Can you work these out from the model? Positions are in its coordinate system, mm. A direction names the side the tool comes from. Give positions to 0.01 mm unless a question says otherwise; leave off trailing zeros. Loops run counter-clockwise (first coordinate to the right, second up) from the corner with the lowest first, then second, coordinate; pieces in that order, holes last. Notation, with made-up numbers: M -19.75,78 L -9.75,78 A12 ccw -9.75,101 Z; hole C -34.75,38 d1. An arc over 180 degrees is marked long. Use CSV: the item, a comma, the result in double quotes.
from build123d import *

# Parameters (mm, degrees)
F1_R           = 1.75
F2_DEPTH       = 5
F3_R           = 1.75
F4_DEPTH       = 5
F6_R           = 25
F7_DEPTH       = 5.001
F9_D           = 3.3
F9_CSINK_D     = 6.72
F9_CSINK_ANGLE = 90
F10_R          = 1.75
F11_DEPTH      = 2.5


with BuildPart() as f2:
    # F1 (on Top) → F2 (new body)
    with BuildSketch(Plane.XY):
        with BuildLine():
            Line((-1.4142135624, 41.0121933088), (-41.0121933088, 1.4142135624))
            ThreePointArc((-41.0121933088, 1.4142135624), (-41.5979797464, 0), (-41.0121933088, -1.4142135624))
            Line((-41.0121933088, -1.4142135624), (-1.4142135624, -41.0121933088))
            ThreePointArc((-1.4142135624, -41.0121933088), (0, -41.5979797464), (1.4142135624, -41.0121933088))
            Line((1.4142135624, -41.0121933088), (41.0121933088, -1.4142135624))
            ThreePointArc((41.0121933088, -1.4142135624), (41.5979797464, 0), (41.0121933088, 1.4142135624))
            Line((41.0121933088, 1.4142135624), (1.4142135624, 41.0121933088))
            ThreePointArc((1.4142135624, 41.0121933088), (0, 41.5979797464), (-1.4142135624, 41.0121933088))
        make_face()
        with Locations((0, -35.3553390593)):
            Circle(F1_R, mode=Mode.SUBTRACT)
        with Locations((-35.3553390593, 0)):
            Circle(F1_R, mode=Mode.SUBTRACT)
        with Locations((35.3553390593, 0)):
            Circle(F1_R, mode=Mode.SUBTRACT)
        with Locations((0, 35.3553390593)):
            Circle(F1_R, mode=Mode.SUBTRACT)
    extrude(amount=F2_DEPTH)


with BuildPart() as f4:
    # F3 (on Top) → F4 (new body)
    with BuildSketch(Plane.XY):
        with BuildLine():
            Line((23, 25), (-23, 25))
            ThreePointArc((-23, 25), (-24.4142135624, 24.4142135624), (-25, 23))
            Line((-25, 23), (-25, -23))
            ThreePointArc((-25, -23), (-24.4142135624, -24.4142135624), (-23, -25))
            Line((-23, -25), (23, -25))
            ThreePointArc((23, -25), (24.4142135624, -24.4142135624), (25, -23))
            Line((25, -23), (25, 23))
            ThreePointArc((25, 23), (24.4142135624, 24.4142135624), (23, 25))
        make_face()
        with Locations((-20, -20)):
            Circle(F3_R, mode=Mode.SUBTRACT)
        with Locations((20, -20)):
            Circle(F3_R, mode=Mode.SUBTRACT)
        with Locations((-20, 20)):
            Circle(F3_R, mode=Mode.SUBTRACT)
        with Locations((20, 20)):
            Circle(F3_R, mode=Mode.SUBTRACT)
    extrude(amount=F4_DEPTH)

    # F5: union F2
    add(f2.part)

    # F6 (on face) → F7 (cut, through all)
    with BuildSketch(Plane.XY.offset(5)):
        Circle(F6_R)
    extrude(amount=-F7_DEPTH, mode=Mode.SUBTRACT)


with BuildPart() as f4_1:
    # F8: moved
    add(f4.part.moved(Location((0, 0, -5))))

    # F9 (through all)
    with Locations(Plane.XY):
        with Locations((-20, -20), (20, 20), (20, -20), (-20, 20)):
            CounterSinkHole(F9_D / 2, F9_CSINK_D / 2, counter_sink_angle=F9_CSINK_ANGLE)

    # F10 (on face) → F11 (cut)
    with BuildSketch(Plane(origin=(0, 0, -5), x_dir=(1, 0, 0), z_dir=(0, 0, -1))):
        Polygon((37.0428390593, 2.9228357378), (33.6678390593, 2.9228357378), (31.9803390593, 0), (33.6678390593, -2.9228357378), (37.0428390593, -2.9228357378), (38.7303390593, 0), align=None)
        with Locations((35.3553390593, 0)):
            Circle(F10_R, mode=Mode.SUBTRACT)
        Polygon((-2.9228357378, 33.6678390593), (0, 31.9803390593), (2.9228357378, 33.6678390593), (2.9228357378, 37.0428390593), (0, 38.7303390593), (-2.9228357378, 37.0428390593), align=None)
        with Locations((0, 35.3553390593)):
            Circle(F10_R, mode=Mode.SUBTRACT)
        Polygon((0, -38.7303390593), (2.9228357378, -37.0428390593), (2.9228357378, -33.6678390593), (0, -31.9803390593), (-2.9228357378, -33.6678390593), (-2.9228357378, -37.0428390593), align=None)
        with Locations((0, -35.3553390593)):
            Circle(F10_R, mode=Mode.SUBTRACT)
        Polygon((-38.7303390593, 0), (-37.0428390593, -2.9228357378), (-33.6678390593, -2.9228357378), (-31.9803390593, 0), (-33.6678390593, 2.9228357378), (-37.0428390593, 2.9228357378), align=None)
        with Locations((-35.3553390593, 0)):
            Circle(F10_R, mode=Mode.SUBTRACT)
    extrude(amount=-F11_DEPTH, mode=Mode.SUBTRACT)


solid = f4_1.part
Q1. I want a section at A-A, the plane x = -20. Please give me the cut outline in (y, z), then the cut area to 3 significant figures.
Model answer:
outline,"M -25,-5 L -21.65,-5 L -21.65,-1.71 L -23.36,0 L -25,0 Z; M -18.35,-5 L -15,-5 L -15,0 L -16.64,0 L -18.35,-1.71 Z; M 15,-5 L 18.35,-5 L 18.35,-1.71 L 16.64,0 L 15,0 Z; M 21.65,-5 L 25,-5 L 25,0 L 23.36,0 L 21.65,-1.71 Z"
area,"61.2 mm2"
Q2. For faces 1 (the flat face through (20, 25, -3)), 2 (the cylindrical face through (-24.4, 24.43, -2.54)), 3 (the flat face through (2.923, 35, -4)), which set-ups out of +Z, -Z, +X, -X, +Y, -Y let a thin tool reach every point of the face, with its end or its side?
Model answer:
face 1,"+Z, -Z, +X, +Y"
face 2,"+Z, -Z, -X, +Y"
face 3,"-Z"
Q3. If we mould it in two halves opening along X, with no side actions, what happens to faces 4 (the flat face through (9.308, -33.118, -2.535)), 5 (the flat face through (-37.9, 1.44, -3.77)), 6 (the cylindrical face through (0.022, 41.598, -2.535))? For each: released by +X, released by -X, zero draft, split by the parting line, or undercut.
Model answer:
face 4,"released by +X"
face 5,"undercut"
face 6,"split by the parting line"
Q4. I want a section at C-C, the plane x = -9.5. Please give me the cut outline in (y, z).
Model answer:
outline,"M -32.93,-5 L -23.12,-5 L -23.12,0 L -32.93,0 Z; M 23.12,-5 L 32.93,-5 L 32.93,0 L 23.12,0 Z"
Q5. Please list where these lines run through material, in increasing order: L1, parallel to Y at x = 0, z = -1.85; L2, parallel to Y at x = -20, z = -3.7. Write a range as from..to.
Model answer:
L1,"-41.6..-37.11, -33.61..-25, 25..33.61, 37.11..41.6"
L2,"-25..-21.65, -18.35..-15, 15..18.35, 21.65..25"
Q6. I want a section at B-B, the plane y = 12. Please give me the cut outline in (x, z).
Model answer:
outline,"M -30.43,-5 L -21.93,-5 L -21.93,0 L -30.43,0 Z; M 21.93,-5 L 30.43,-5 L 30.43,0 L 21.93,0 Z"
Q7. I'm going to push flat-ended pins straight in: P1, Ø3, axis at x = 20, y = 20, coming from the +Z side; P2, Ø1.5, axis at x = 20.5, z = -2, coming from the -Y side; P3, Ø1.2, axis at y = 35.5, z = -4, coming from the -X side; P4, Ø2.5, axis at y = -21, z = -3.5, coming from the +X side. Where does each tip first touch, or does it pass through?
Model answer:
P1,"through"
P2,"y = -25"
P3,"x = -7.53"
P4,"x = 25"
Q8. I want a section at D-D, the plane z = -4.1. State how many separate pieces and enclosed holes the cut face has, then the cut area to 3 significant figures.
Model answer:
separate pieces,"1"
enclosed holes,"13"
area,"1,590 mm2"
